Here's how the part is built. I have some questions about the finished solid (model axes, mm). A direction names the side the tool comes from. Coordinates: 2 decimals unless noted, no trailing zeros. Write each loop counter-clockwise with the first axis right and the second up, starting at its lowest first coordinate (ties: lowest second). Pieces come first, ordered by that corner, then holes. Notation, with made-up numbers: M -37.5,67 L 7.5,67 A17 ccw 7.5,72 Z; hole C 74.5,83.25 d11. An arc over 180 degrees is marked long. Use a Markdown table: item, result.
```python
from build123d import *

# Parameters (mm, degrees)
F3_DEPTH = 4
F4_SIZE  = 1


with BuildPart() as f1:
    # F0 (on Front) → F1 (revolve)
    with BuildSketch(Plane.XZ):
        Polygon((5, 6), (0, 6), (0, -50), (3, -50), (3, 0), (5, 0), align=None)
    revolve(axis=Axis((0, 0, -50.553678), (0, 0, -1)))

    # F2 (on face) → F3 (cut)
    with BuildSketch(Plane.XY.offset(6)):
        Polygon((1.443376, 2.5), (-1.443376, 2.5), (-2.886751, 0), (-1.443376, -2.5), (1.443376, -2.5), (2.886751, 0), align=None)
    extrude(amount=-F3_DEPTH, mode=Mode.SUBTRACT)

    # F4
    f4_edges = [f1.edges().sort_by_distance(p)[0] for p in [
        (-3, 0, -50),
    ]]
    chamfer(f4_edges, length=F4_SIZE)


solid = f1.part
```
1. I need wall thicknesses on probe 1 along X at (y, z) = (0.25, -44.5); probe 2 along Z at (x, y) = (0, -1.25); probe 3 along Z at (x, y) = (-2, 3.25). Which ranges of each line are inside material? Lowest first, please.
Answers follow:
| item | result |
|---|---|
| probe 1 | x = -2.99 to 2.99 |
| probe 2 | z = -50 to 2 |
| probe 3 | z = 0 to 6 |
2. We'd pull the mould along X, two halves only. Please class faces 1 (the face through (2.155, -1.267, 4.028)), 2 (the face through (-1.08, 4.88, 3.04)), 3 (the face through (-3.3, -0.1, 0)): +X half, -X half, draft (parallel to the pull), parting line (faces both ways), or undercut.
Answers follow:
| item | result |
|---|---|
| face 1 | undercut |
| face 2 | parting line |
| face 3 | draft |
3. Will these pins go through, and if not, where does the flat tip stop? pin 1 Ø1 at (x, y) = (-3.5, -1) entering from -Z; pin 2 Ø4 at (y, z) = (-1, -33) entering from -X; pin 3 Ø1 at (y, z) = (-0.5, -4) entering from +X.
Answers follow:
| item | result |
|---|---|
| pin 1 | stops at z = 0 |
| pin 2 | stops at x = -3 |
| pin 3 | stops at x = 3 |
4. Suppose I cut it at D-D on x = 3.5. Write out the boundary of the cut face in (y, z), and give its area (3 significant figures).
Answers follow:
| item | result |
|---|---|
| outline | M -3.57,0 L 3.57,0 L 3.57,6 L -3.57,6 Z |
| area | 42.8 mm2 |
5. Suppose I cut it at C-C on y = 3.75. Write out the boundary of the cut face in (x, z), and give its area (3 significant figures).
Answers follow:
| item | result |
|---|---|
| outline | M -3.31,0 L 3.31,0 L 3.31,6 L -3.31,6 Z |
| area | 39.7 mm2 |
6. Which directions (+Z, -Z, +X, -X, +Y, -Y) give clear straight access to the entire face, cutting with the end or side of a thin tool? Please do faces 4 (the face through (2, 2, 6)), 5 (the face through (-3, 0, -24)), 6 (the face through (0, 0, 2)).
Answers follow:
| item | result |
|---|---|
| face 4 | +Z, +X, -X, +Y, -Y |
| face 5 | -Z |
| face 6 | +Z |
7. Suppose I cut it at B-B on z = -6. Write out the boundary of the cut face in (x, y).
Answers follow:
| item | result |
|---|---|
| outline | C 0,0 d6 |
8. Suppose I cut it at A-A on x = 0. Write out the boundary of the cut face in (y, z).
Answers follow:
| item | result |
|---|---|
| outline | M -5,0 L -3,0 L -3,-49 L -2,-50 L 2,-50 L 3,-49 L 3,0 L 5,0 L 5,6 L 2.5,6 L 2.5,2 L -2.5,2 L -2.5,6 L -5,6 Z |
